Geometry: final body of the model. Coordinates: model frame, mm. A direction names the side the tool comes from. Round coordinates to 2 decimals unless told otherwise and drop trailing zeros. Loops run counter-clockwise (first coordinate to the right, second up) from the corner with the lowest first, then second, coordinate; pieces in that order, holes last. Notation, with made-up numbers: (75, 55.25) - (122, 55.25) arc R15 cw to (122, 76.25) - close; hole circle Ø5 at (-30.75, 45.25). An arc over 180 degrees is marked (long way). Answer as CSV lines item,"result".
from build123d import *

# Parameters (mm, degrees)
REVOLVE1_ANGLE                                       = 180
SKETCH2_W                                            = 3
SKETCH2_H                                            = 20
BOSS_EXTRUDE1_DEPTH                                  = 10
SKETCH4_W                                            = 1
SKETCH4_H                                            = 20
CUT_EXTRUDE1_DEPTH                                   = 0.01
CSK_FOR_M1_6_COUNTERSUNK_FLAT_HEAD_SCREW_D           = 1.8
CSK_FOR_M1_6_COUNTERSUNK_FLAT_HEAD_SCREW_DEPTH       = 5
CSK_FOR_M1_6_COUNTERSUNK_FLAT_HEAD_SCREW_CSINK_D     = 3.6
CSK_FOR_M1_6_COUNTERSUNK_FLAT_HEAD_SCREW_CSINK_ANGLE = 90
CSK_FOR_M1_6_COUNTERSUNK_FLAT_HEAD_SCREW_TIP         = 0.540774557
CSK_FOR_M1_6_COUNTERSUNK_FLAT_HEAD_S_2_D             = 1.8
CSK_FOR_M1_6_COUNTERSUNK_FLAT_HEAD_S_2_DEPTH         = 5
CSK_FOR_M1_6_COUNTERSUNK_FLAT_HEAD_S_2_CSINK_D       = 3.6
CSK_FOR_M1_6_COUNTERSUNK_FLAT_HEAD_S_2_CSINK_ANGLE   = 90
CSK_FOR_M1_6_COUNTERSUNK_FLAT_HEAD_S_2_TIP           = 0.540774557
CSK_FOR_M1_6_COUNTERSUNK_FLAT_HEAD_S_3_D             = 1.8
CSK_FOR_M1_6_COUNTERSUNK_FLAT_HEAD_S_3_DEPTH         = 5
CSK_FOR_M1_6_COUNTERSUNK_FLAT_HEAD_S_3_CSINK_D       = 3.6
CSK_FOR_M1_6_COUNTERSUNK_FLAT_HEAD_S_3_CSINK_ANGLE   = 90
CSK_FOR_M1_6_COUNTERSUNK_FLAT_HEAD_S_3_TIP           = 0.540774557
SKETCH10_W                                           = 1
SKETCH10_H                                           = 20
BOSS_EXTRUDE2_DEPTH                                  = 10.01
SKETCH12_R                                           = 3
CUT_EXTRUDE4_DEPTH                                   = 3
CUT_EXTRUDE5_START                                   = -3
SKETCH13_R                                           = 3
CUT_EXTRUDE5_DEPTH                                   = 3


with BuildPart() as part:
    # Sketch1 → Revolve1 (revolve)
    with BuildSketch(Plane.XY):
        with BuildLine():
            Line((61, 170), (61, 0))
            Line((61, 0), (58, 0))
            Line((58, 0), (58, 170))
            ThreePointArc((58, 170), (41.873834296, 218.154039035), (0, 246.884627213))
            Line((0, 246.884627213), (0, 250))
            ThreePointArc((0, 250), (44.010282534, 220.301590432), (61, 170))
        make_face()
    revolve(axis=Axis((0, 0, 0), (0, 1, 0)), revolution_arc=REVOLVE1_ANGLE)

    # Sketch2 → Boss-Extrude1 (add)
    with BuildSketch(Plane.XY):
        with Locations((56.5, 152)):
            Rectangle(SKETCH2_W, SKETCH2_H)
        with Locations((-56.5, 152)):
            Rectangle(SKETCH2_W, SKETCH2_H)
    extrude(amount=-BOSS_EXTRUDE1_DEPTH)

    # Sketch4 → Cut-Extrude1 (cut)
    with BuildSketch(Plane.XY):
        with Locations((-56.5, 152)):
            Rectangle(SKETCH4_W, SKETCH4_H)
        with Locations((56.5, 152)):
            Rectangle(SKETCH4_W, SKETCH4_H)
    extrude(amount=-CUT_EXTRUDE1_DEPTH, mode=Mode.SUBTRACT)

    # CSK for M1.6 Countersunk Flat Head Screw2
    with Locations(Plane(origin=(60.795081967, 157.001615154, -4.995799095), x_dir=(0.081898345823, 0, 0.996640687987), z_dir=(0.996640687987, 0, -0.081898345823))):
        with Locations((0, 0)):
            CounterSinkHole(CSK_FOR_M1_6_COUNTERSUNK_FLAT_HEAD_SCREW_D / 2, CSK_FOR_M1_6_COUNTERSUNK_FLAT_HEAD_SCREW_CSINK_D / 2, depth=CSK_FOR_M1_6_COUNTERSUNK_FLAT_HEAD_SCREW_DEPTH, counter_sink_angle=CSK_FOR_M1_6_COUNTERSUNK_FLAT_HEAD_SCREW_CSINK_ANGLE)
            with Locations((0, 0, -(CSK_FOR_M1_6_COUNTERSUNK_FLAT_HEAD_SCREW_DEPTH + CSK_FOR_M1_6_COUNTERSUNK_FLAT_HEAD_SCREW_TIP / 2))):  # 118° drill point
                Cone(0, CSK_FOR_M1_6_COUNTERSUNK_FLAT_HEAD_SCREW_D / 2, CSK_FOR_M1_6_COUNTERSUNK_FLAT_HEAD_SCREW_TIP, mode=Mode.SUBTRACT)

    # CSK for M1.6 Countersunk Flat Head S 2
    with Locations(Plane(origin=(60.795081967, 147.001615154, -4.995799095), x_dir=(0.081897976852, 0, 0.996640718307), z_dir=(0.996640718307, 0, -0.081897976852))):
        with Locations((0, 0)):
            CounterSinkHole(CSK_FOR_M1_6_COUNTERSUNK_FLAT_HEAD_S_2_D / 2, CSK_FOR_M1_6_COUNTERSUNK_FLAT_HEAD_S_2_CSINK_D / 2, depth=CSK_FOR_M1_6_COUNTERSUNK_FLAT_HEAD_S_2_DEPTH, counter_sink_angle=CSK_FOR_M1_6_COUNTERSUNK_FLAT_HEAD_S_2_CSINK_ANGLE)
            with Locations((0, 0, -(CSK_FOR_M1_6_COUNTERSUNK_FLAT_HEAD_S_2_DEPTH + CSK_FOR_M1_6_COUNTERSUNK_FLAT_HEAD_S_2_TIP / 2))):  # 118° drill point
                Cone(0, CSK_FOR_M1_6_COUNTERSUNK_FLAT_HEAD_S_2_D / 2, CSK_FOR_M1_6_COUNTERSUNK_FLAT_HEAD_S_2_TIP, mode=Mode.SUBTRACT)

    # CSK for M1.6 Countersunk Flat Head S 3
    with Locations(Plane(origin=(-60.795081967, 147.001615154, -4.995799095), x_dir=(0.081897976852, 0, -0.996640718307), z_dir=(-0.996640718307, 0, -0.081897976852))):
        with Locations((0, 0), (0, -10)):
            CounterSinkHole(CSK_FOR_M1_6_COUNTERSUNK_FLAT_HEAD_S_3_D / 2, CSK_FOR_M1_6_COUNTERSUNK_FLAT_HEAD_S_3_CSINK_D / 2, depth=CSK_FOR_M1_6_COUNTERSUNK_FLAT_HEAD_S_3_DEPTH, counter_sink_angle=CSK_FOR_M1_6_COUNTERSUNK_FLAT_HEAD_S_3_CSINK_ANGLE)
            with Locations((0, 0, -(CSK_FOR_M1_6_COUNTERSUNK_FLAT_HEAD_S_3_DEPTH + CSK_FOR_M1_6_COUNTERSUNK_FLAT_HEAD_S_3_TIP / 2))):  # 118° drill point
                Cone(0, CSK_FOR_M1_6_COUNTERSUNK_FLAT_HEAD_S_3_D / 2, CSK_FOR_M1_6_COUNTERSUNK_FLAT_HEAD_S_3_TIP, mode=Mode.SUBTRACT)

    # Sketch10 → Boss-Extrude2 (add)
    with BuildSketch(Plane.XY.offset(-0.01)):
        with Locations((-55.5, 152)):
            Rectangle(SKETCH10_W, SKETCH10_H)
        with Locations((55.5, 152)):
            Rectangle(SKETCH10_W, SKETCH10_H)
    extrude(amount=BOSS_EXTRUDE2_DEPTH)

    # Sketch12 → Cut-Extrude4 (cut)
    with BuildSketch(Plane(origin=(-55, 0, 0), x_dir=(0, 0, -1), z_dir=(1, 0, 0))):
        with Locations((0, 152)):
            Circle(SKETCH12_R)
    extrude(amount=-CUT_EXTRUDE4_DEPTH, mode=Mode.SUBTRACT)

    # Sketch13 → Cut-Extrude5 (cut)
    with BuildSketch(Plane.ZY.offset(-55).offset(CUT_EXTRUDE5_START)):
        with Locations(Location((0, 152, 0), (0, 0, 180))):
            Circle(SKETCH13_R)
    extrude(amount=CUT_EXTRUDE5_DEPTH, mode=Mode.SUBTRACT)


solid = part.part
(1) Pin query (flat end, axial travel): P1, Ø4, axis at x = -22.5, y = 101, coming from the +Z side; P2, Ø2.5, axis at x = 56, z = 2, coming from the -Y side; P3, Ø0.5, axis at x = 56.5, y = 145.5, coming from the +Z side. Return the tip coordinate at first contact, or that it passes through.
Findings below:
P1,"z = -52.57"
P2,"y = 142"
P3,"z = -0.01"
(2) Material intervals for line 1 along X through (y, z) = (111, -10.5); line 2 along X through (y, z) = (112.5, -19.5); line 3 along Y through (x, z) = (-44, -8), sorted ascending.
Findings below:
line 1,"-60.09 to -57.04, 57.04 to 60.09"
line 2,"-57.8 to -54.62, 54.62 to 57.8"
line 3,"214.13 to 219.36"
(3) Draft query along Y for faces 1 (the face through (56, 152, 5)), 2 (the face through (-56.15, 150.85, -2.77)), 3 (the face through (9, 0, -58)). Return one class per face: pulls with the +Y half, pulls with the -Y half, needs draft (parallel to the pull), parting line crosses it, or undercut.
Findings below:
face 1,"needs draft"
face 2,"undercut"
face 3,"pulls with the -Y half"
(4) Section A-A (y = 152). Output: boundary loops of the cut face in (x, z).
Findings below:
outline,"(-61, 0) arc R61 ccw to (61, 0) - (58, 0) - (58, -3) - (55, -3) - (55, -10) - (57.13, -10) arc R58 cw to (-57.13, -10) - (-55, -10) - (-55, -3) - (-58, -3) - (-58, 0) - close; (-56, 3) - (-55, 3) - (-55, 10) - (-56, 10) - close; (55, 3) - (56, 3) - (56, 10) - (55, 10) - close"
(5) Access query for faces 4 (the face through (-55, 149.6, -2.4)), 5 (the face through (1.341, 83.81, -60.985)), 6 (the face through (56.19, 153.15, -2.77)). Directions: +Z, -Z, +X, -X, +Y, -Y. A direction counts if a zero-diameter tool reaches every point of the face in a straight line with its end or side. Return the directions, or none.
Findings below:
face 4,"+Z, -Y"
face 5,"-Z, +Y, -Y"
face 6,"none"
